Drawing for the job (mm, zero at the part's lowest x, y, z). Give positions to 0.01 mm unless a question says otherwise; leave off trailing zeros. Write each loop counter-clockwise with the first axis right and the second up, starting at its lowest first coordinate (ties: lowest second). Pieces come first, ordered by that corner, then holes.
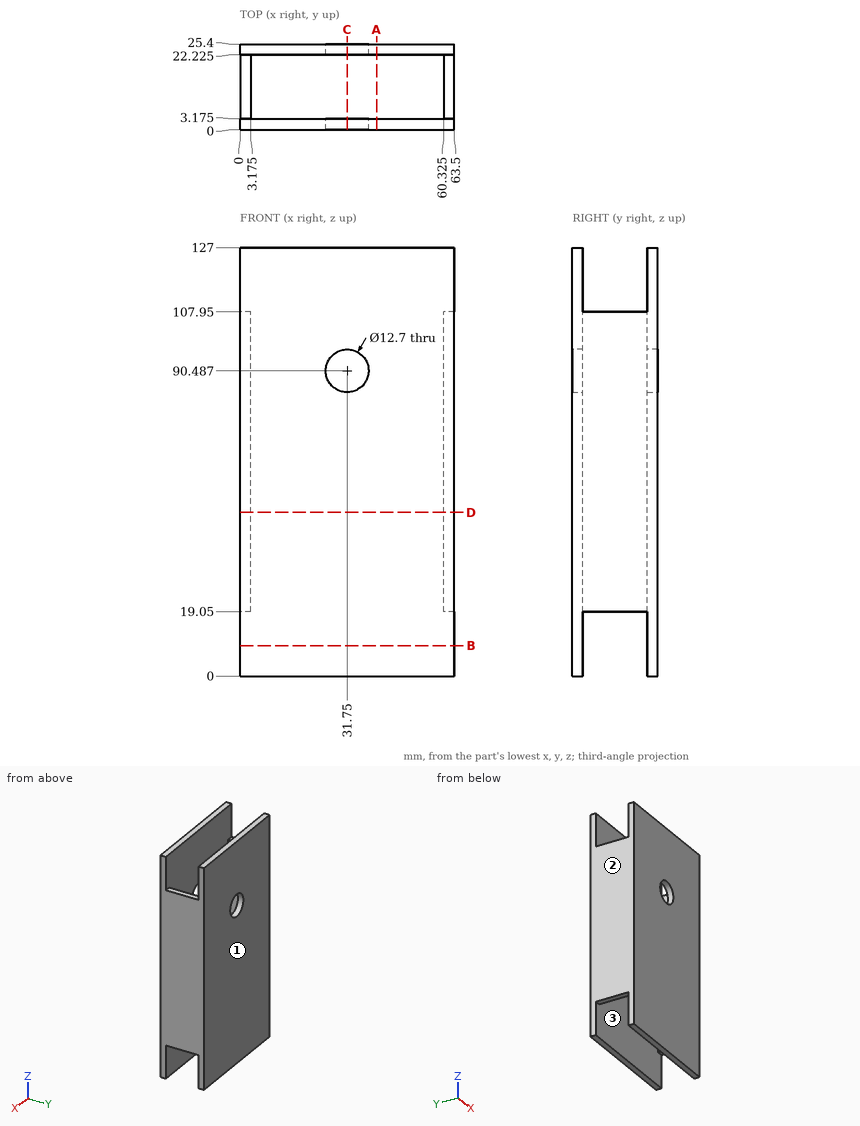
1. Pull direction X, two halves, no side cores. Call the marked faces 1, 2 and 3: +X half, -X half, draft (parallel to the pull), parting line (faces both ways), or undercut.
Calculated:
face 1: draft
face 2: -X half
face 3: undercut
2. Pin check, flat tips, straight feed: P1, Ø1.6, axis at x = 1, y = 10.5, coming from the -Z side; P2, Ø2.5, axis at x = 62.5, y = 15, coming from the +Z side; P3, Ø1.5, axis at x = 40.5, y = 19.5, coming from the +Z side. Stop position of each tip, or through.
Calculated:
P1: stops at z = 19.05
P2: stops at z = 107.95
P3: passes through
3. Slice it at D-D, the plane z = 48.5. Write the cut outline in (x, y) (1 decimal).
Calculated:
outline: (0, 0) - (63.5, 0) - (63.5, 25.4) - (0, 25.4) - close; hole (3.2, 3.2) - (60.3, 3.2) - (60.3, 22.2) - (3.2, 22.2) - close
4. Slice it at C-C, the plane x = 31.75. Write the cut outline in (y, z) (1 decimal).
Calculated:
outline: (0, 0) - (3.2, 0) - (3.2, 84.1) - (0, 84.1) - close; (0, 96.8) - (3.2, 96.8) - (3.2, 127) - (0, 127) - close; (22.2, 0) - (25.4, 0) - (25.4, 84.1) - (22.2, 84.1) - close; (22.2, 96.8) - (25.4, 96.8) - (25.4, 127) - (22.2, 127) - close
5. Slice it at B-B, the plane z = 9. Write the cut outline in (x, y) (1 decimal).
Calculated:
outline: (0, 0) - (63.5, 0) - (63.5, 3.2) - (0, 3.2) - close; (0, 22.2) - (63.5, 22.2) - (63.5, 25.4) - (0, 25.4) - close
6. Slice it at A-A, the plane x = 40.5. Write the cut outline in (y, z) (1 decimal).
Calculated:
outline: (0, 0) - (3.2, 0) - (3.2, 127) - (0, 127) - close; (22.2, 0) - (25.4, 0) - (25.4, 127) - (22.2, 127) - close
7. Probe probe 1 along X at (y, z) = (8.5, 51) (1 decimal); probe 2 along Y at (x, z) = (18.5, 86) (1 decimal). List the from-to ranges inside material, lowest first.
Calculated:
probe 1: x = 0 to 3.2, 60.3 to 63.5
probe 2: y = 0 to 3.2, 22.2 to 25.4
